Build history of the part. All positions in model axes, mm. A direction names the side the tool comes from. Round coordinates to 2 decimals unless told otherwise and drop trailing zeros. Write each loop counter-clockwise with the first axis right and the second up, starting at its lowest first coordinate (ties: lowest second). Pieces come first, ordered by that corner, then holes. Notation, with made-up numbers: M 69,33.5 L 118,33.5 A14 cw 118,58.5 Z; hole C -4,-31 d9. An arc over 180 degrees is marked long. Write item = value, one per line.
Autodesk Inventor part; units mm, degrees
ref_plane "YZ Plane" through (0, 0, 0) normal (1, 0, 0) x (0, 1, 0)
ref_plane "XZ Plane" through (0, 0, 0) normal (0, 1, 0) x (-1, 0, 0)
ref_plane "XY Plane" through (0, 0, 0) normal (0, 0, 1) x (1, 0, 0)
sketch "Sketch1" plane through (0, 0, 0) normal (0, 1, 0) x (-1, 0, 0)
  line L0 (-4, 4.05) -> (4, 4.05)
  line L1 (4, 4.05) -> (4, -4.05)
  line L2 (4, -4.05) -> (-4, -4.05)
  line L3 (-4, -4.05) -> (-4, 4.05)
  line L4 (-4, 4.05) -> (4, -4.05) construction
  line L5 (4, 4.05) -> (-4, -4.05) construction
  line L6 (8, 6.05) -> (-5, 6.05)
  line L7 (-5, 6.05) -> (-5, -6.05)
  line L8 (-5, -6.05) -> (8, -6.05)
  line L9 (8, -6.05) -> (8, 6.05)
  point P0 (0, 0)
  dimension "d0" = 8.1
  dimension "d1" = 8
  dimension "d5" = 2
  dimension "d6" = 2
  dimension "d7" = 1
  dimension "d8" = 4
extrude "Extrusion1" add sketch "Sketch1" along normal blind 5
sketch "Sketch2" plane through (0, 0, 0) normal (0, -1, 0) x (1, 0, 0)
  line L0 (5, 6.05) -> (5, -6.05)
  line L1 (-8, 6.05) -> (5, 6.05)
  line L2 (-8, -6.05) -> (-8, 6.05)
  line L3 (5, -6.05) -> (-8, -6.05)
  line L4 (4, 4.05) -> (-4, 4.05)
  line L5 (4, -4.05) -> (4, 4.05)
  line L6 (-4, -4.05) -> (4, -4.05)
  line L7 (-4, 4.05) -> (-4, -4.05)
  point P0 (0, 0)
extrude "Extrusion2" add sketch "Sketch2" along normal blind 4 contours L0 L3 L2 L1 | L5 L6 L7 L4
sketch "Sketch3" plane through (0, 5, 0) normal (0, 1, 0) x (1, 0, 0)
  line L0 (-4, -4.05) -> (-4, 4.05)
  circle A0 centre (-4.8, 0) radius 0.8
  point P0 (0, 0)
  dimension "d14" = 1.6
extrude "Extrusion3" cut sketch "Sketch3" against normal blind 100
sketch "Sketch4" plane through (0, 0, 0) normal (0, 1, 0) x (1, 0, 0)
  line L0 (-0.2, -2.5) -> (-2.2, -2.5)
  line L1 (-2.2, -2.5) -> (-2.2, 2.5)
  line L2 (-2.2, 2.5) -> (-0.2, 2.5)
  line L3 (-0.2, 2.5) -> (-0.2, -2.5)
  line L4 (-0.2, -2.5) -> (-2.2, 2.5) construction
  line L5 (-2.2, -2.5) -> (-0.2, 2.5) construction
  line L6 (-4, -4.05) -> (-4, 0)
  point P0 (0, 0)
  point P1 (-1.2, 0)
  point P2 (-1.2, 0)
  dimension "d17" = 5
  dimension "d18" = 3.8
  dimension "d19" = 2
extrude "Extrusion4" cut sketch "Sketch4" against normal blind 100
fillet "Fillet1" radius 2 11 edges at (-8, 0.5, -6.05) (5, 0.5, -6.05) (-8, 0.5, 6.05) (5, 0.5, 6.05) (-1.5, -4, 6.05) (-8, -4, 0) (-1.5, -4, -6.05) (-1.5, 5, 6.05) (-8, 5, 0) (-1.5, 5, -6.05) (5, -4, 0)
properties part number "Cable_tie_connector_p1"
1. Mould opens along X. For faces 4 (the face through (4.43, -3.4, -0.06)), 5 (the face through (-0.58, 4.43, -5.45)), 6 (the face through (-5.43, 0.56, 0.49)) say: pulls with the +X half, pulls with the -X half, needs draft (parallel to the pull), parting line crosses it, or undercut.
Responses:
face_4 = pulls with the +X half
face_5 = needs draft
face_6 = undercut
2. Probe probe 1 along X at (y, z) = (-0.5, 0); probe 2 along X at (y, z) = (0.5, 1.5); probe 3 along Z at (x, y) = (-4.8, -0.25). List the from-to ranges inside material, lowest first.
Responses:
probe_1 = -8 to -5.6, -4 to -2.2, -0.2 to 5
probe_2 = -8 to -4, 4 to 5
probe_3 = -6.05 to -0.8, 0.8 to 6.05
3. Band-saw the part on B-B (y = -1.25). List the corners of the cut face in (x, z).
Responses:
outline = M -8,-4.05 A2 ccw -6,-6.05 L 3,-6.05 A2 ccw 5,-4.05 L 5,4.05 A2 ccw 3,6.05 L -6,6.05 A2 ccw -8,4.05 Z; hole C -4.8,0 d1.6; hole M -2.2,-2.5 L -0.2,-2.5 L -0.2,2.5 L -2.2,2.5 Z
4. Tool access for faces 1 (the face through (0, 2, -4.05)), 2 (the face through (-7.43, 0.46, -5.45)), 3 (the face through (-2.2, -2, 0)): list every direction of +Z, -Z, +X, -X, +Y, -Y with a clear straight run to the whole face (end or side of a thin tool).
Responses:
face_1 = +Y
face_2 = -Z, -X, +Y, -Y
face_3 = +Y, -Y
5. Flat gauge pins, fed straight in: pin 1 (4.5 mm diameter, centred on y = -2.5, z = 0, fed in from -X); pin 2 (2.5 mm diameter, centred on x = 1.5, z = -1, fed in from +Y). Where does each tip first touch, or does it go through?
Responses:
pin_1 = -8
pin_2 = 0
6. Band-saw the part on A-A (x = -4.8). List the corners of the cut face in (y, z).
Responses:
outline = M -4,-4.05 A2 ccw -2,-6.05 L 3,-6.05 A2 ccw 5,-4.05 L 5,-0.8 L -4,-0.8 Z; M -4,0.8 L 5,0.8 L 5,4.05 A2 ccw 3,6.05 L -2,6.05 A2 ccw -4,4.05 Z
